```python
from build123d import *

# Parameters (mm, degrees)
F1_DEPTH = 25
F2_T     = -1


with BuildPart() as f1:
    # F0 (on Top) → F1 (new body)
    with BuildSketch(Plane.XY):
        Polygon((35.2, 26.95), (35.2, 29.45), (-35.2, 29.45), (-35.2, 26.95), (-37.7, 26.95), (-37.7, -26.95), (-35.2, -26.95), (-35.2, -29.45), (35.2, -29.45), (35.2, -26.95), (37.7, -26.95), (37.7, 26.95), align=None)
    extrude(amount=F1_DEPTH)

    # F2
    f2_openings = [f1.faces().sort_by_distance(p)[0] for p in [
        (0, 0, 25),
    ]]
    offset(amount=F2_T, openings=f2_openings, kind=Kind.INTERSECTION)


solid = f1.part
```
Design review of the part built by this model. Coordinates are the model's own, in mm. A direction names the side the tool comes from. Coordinates: 2 decimals unless noted, no trailing zeros. Write each loop counter-clockwise with the first axis right and the second up, starting at its lowest first coordinate (ties: lowest second). Pieces come first, ordered by that corner, then holes.
1) To check wall thickness, follow L1, parallel to Y at x = -25.5, z = 7.5; L2, parallel to X at y = 13, z = 23.5; L3, parallel to X at y = -27, z = 6.75. State the ranges of each line that lie inside material, in increasing order.
2) Insertion check: pin 1 (6 mm diameter, centred on x = 20.5, y = 22.5, fed in from +Z); pin 2 (0.8 mm diameter, centred on x = -36.5, z = 16.5, fed in from +Y); pin 3 (0.8 mm diameter, centred on x = -36, z = 17.5, fed in from -Y). Each pin has a flat end and moves straight along its axis. Give the tip position at first contact, or say it passes through.
3) Machinability: for faces 1 (the flat face through (-35.2, -28, 12)), 2 (the flat face through (-35.2, 28, 12)), 3 (the flat face through (36, -26.95, 12)), 4 (the flat face through (0, -29.45, 12)), 5 (the flat face through (36.7, 0, 13)), which of the approach directions +Z, -Z, +X, -X, +Y, -Y give a long, thin tool a straight path to every point of the face, cutting with its end or side? Answer none if there is none.
4) Add section A-A (z = 6.25). Write out the cut boundary in (x, y).
5) Mouldability with a two-part tool opening along Y and no side actions: class faces 6 (the flat face through (-35, -25.95, 13)), 7 (the flat face through (36, 26.95, 12)), 8 (the flat face through (-37.7, 0, 12)) as +Y half, -Y half, draft (parallel to the pull), parting line (faces both ways), or undercut.
6) Add section C-C (y = -7.5). Write out the cut boundary in (x, z).
7) Add section B-B (x = 4.5). Write out the cut boundary in (y, z), plus the area to 3 significant figures.
Check result:
1. L1: y = -29.45 to -28.45, 28.45 to 29.45
1. L2: x = -37.7 to -36.7, 36.7 to 37.7
1. L3: x = -35.2 to -34.2, 34.2 to 35.2
2. pin 1: stops at z = 1
2. pin 2: stops at y = 26.95
2. pin 3: stops at y = -26.95
3. face 1: +Z, -Z, -X, -Y
3. face 2: +Z, -Z, -X, +Y
3. face 3: +Z, -Z, +X, -Y
3. face 4: +Z, -Z, +X, -X, -Y
3. face 5: +Z
4. outline: (-37.7, -26.95) - (-35.2, -26.95) - (-35.2, -29.45) - (35.2, -29.45) - (35.2, -26.95) - (37.7, -26.95) - (37.7, 26.95) - (35.2, 26.95) - (35.2, 29.45) - (-35.2, 29.45) - (-35.2, 26.95) - (-37.7, 26.95) - close; hole (-36.7, -25.95) - (-34.2, -25.95) - (-34.2, -28.45) - (34.2, -28.45) - (34.2, -25.95) - (36.7, -25.95) - (36.7, 25.95) - (34.2, 25.95) - (34.2, 28.45) - (-34.2, 28.45) - (-34.2, 25.95) - (-36.7, 25.95) - close
5. face 6: undercut
5. face 7: +Y half
5. face 8: draft
6. outline: (-37.7, 0) - (37.7, 0) - (37.7, 25) - (36.7, 25) - (36.7, 1) - (-36.7, 1) - (-36.7, 25) - (-37.7, 25) - close
7. outline: (-29.45, 0) - (29.45, 0) - (29.45, 25) - (28.45, 25) - (28.45, 1) - (-28.45, 1) - (-28.45, 25) - (-29.45, 25) - close
7. area: 107 mm2
